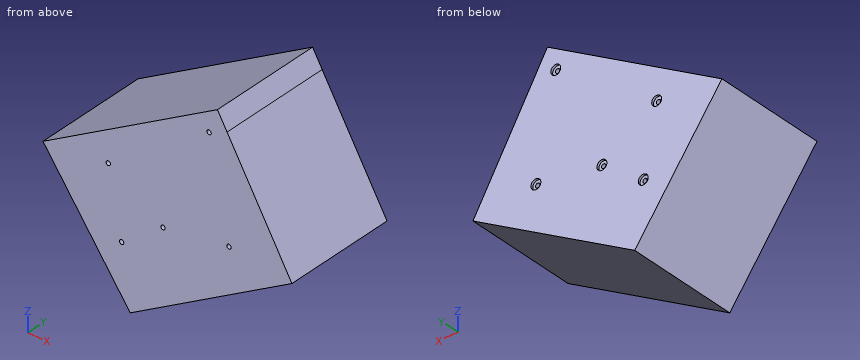
```python
from build123d import *

# Parameters (mm, degrees)
BOSS_EXTRUDE1_DEPTH                                 = 37
CBORE_FOR_00_BINDING_HEAD_MACHINE_SCREW_D           = 1.397
CBORE_FOR_00_BINDING_HEAD_MACHINE_SCREW_CBORE_D     = 3.175
CBORE_FOR_00_BINDING_HEAD_MACHINE_SCREW_CBORE_DEPTH = 0.7112


with BuildPart() as part:
    # Sketch1 → Boss-Extrude1 (new body)
    with BuildSketch(Plane(origin=(0, 0, 0), x_dir=(1, 0, 0), z_dir=(0, 1, 0))):
        Polygon((-10.505392469, 53.079063556), (-38.479053813, 14.047908535), (17.468268874, -18.201203232), (20.541085549, -12.870331878), (41.33210383, 23.198934685), align=None)
    extrude(amount=BOSS_EXTRUDE1_DEPTH)

    # CBORE for #00 Binding Head Machine Screw1 (through all)
    with Locations(Plane(origin=(0, 37, 0), x_dir=(1, 0, 0), z_dir=(0, 1, 0))):
        with Locations((14.7823041, -10.442137487), (0, 23.641654167), (21.162859004, 20.630300354), (-17.558591277, 11.907077475), (-13.254255948, 33.366792883)):
            CounterBoreHole(CBORE_FOR_00_BINDING_HEAD_MACHINE_SCREW_D / 2, CBORE_FOR_00_BINDING_HEAD_MACHINE_SCREW_CBORE_D / 2, CBORE_FOR_00_BINDING_HEAD_MACHINE_SCREW_CBORE_DEPTH)


solid = part.part
```
Geometry: final body of the model. Coordinates: model frame, mm. Give positions to 0.01 mm unless a question says otherwise; leave off trailing zeros. Write each loop counter-clockwise with the first axis right and the second up, starting at its lowest first coordinate (ties: lowest second). Pieces come first, ordered by that corner, then holes.
1. Section query C-C, the plane x = -5. Return loops of the section in (y, z).
2. Section query A-A, the plane y = 34.5. Return loops of the section in (x, z).
3. Section query B-B, the plane z = -46.5. Return loops of the section in (x, y).
4. Line query: probe 1 along Z at (x, y) = (14.5, 25); probe 2 along X at (y, z) = (2, 13.5); probe 3 along Z at (x, y) = (32, 25.5). Output: solid intervals per line, ascending.
5. Pin query (flat end, axial travel): P1, Ø2, axis at x = -27, y = 28.5, coming from the -Z side; P2, Ø2, axis at y = 27.5, z = -15.5, coming from the +X side; P3, Ø1.5, axis at y = 15, z = -18, coming from the -X side. Return the tip coordinate at first contact, or that it passes through.
Computed:
1. outline: (0, -49.91) - (37, -49.91) - (37, 5.25) - (0, 5.25) - close
2. outline: (-38.48, -14.05) - (-10.51, -53.08) - (41.33, -23.2) - (17.47, 18.2) - close; hole circle Ø1.4 at (-17.56, -11.91); hole circle Ø1.4 at (-13.25, -33.37); hole circle Ø1.4 at (0, -23.64); hole circle Ø1.4 at (14.78, 10.44); hole circle Ø1.4 at (21.16, -20.63)
3. outline: (-15.22, 0) - (0.91, 0) - (0.91, 37) - (-15.22, 37) - close
4. probe 1: z = -38.67 to 9.8, 11.08 to 16.49
4. probe 2: x = 9.31 to 20.18
4. probe 3: z = -28.58 to -7.01
5. P1: stops at z = -31.46
5. P2: stops at x = 37.47
5. P3: stops at x = -36.18
